The model under review builds one solid part; all positions refer to its coordinate system, in mm. Face numbers are marked on the shaded views. Give positions to 0.01 mm unless a question says otherwise; leave off trailing zeros. Loops run counter-clockwise (first coordinate to the right, second up) from the corner with the lowest first, then second, coordinate; pieces in that order, holes last. Notation, with made-up numbers: (43.5, -3.75) - (70.5, -3.75) arc R23 ccw to (70.5, 14.25) - close; hole circle Ø6 at (39, 7.25). An arc over 180 degrees is marked (long way). Return JSON: item names as keys, results as strings. Group by question number.
from build123d import *

# Parameters (mm, degrees)
BOSS_EXTRUDE2_DEPTH                        = 12.7
F_13_32_0_40625_DIAMETER_HOLE3_D           = 10.31875
F_13_32_0_40625_DIAMETER_HOLE3_CSINK_D     = 11.58875
F_13_32_0_40625_DIAMETER_HOLE3_CSINK_ANGLE = 90
F_13_32_0_40625_DIAMETER_HOLE2_D           = 10.31875
F_13_32_0_40625_DIAMETER_HOLE2_CSINK_D     = 11.58875
F_13_32_0_40625_DIAMETER_HOLE2_CSINK_ANGLE = 90


with BuildPart() as part:
    # Sketch1 → Boss-Extrude2 (new body)
    with BuildSketch(Plane(origin=(0, 0, 0), x_dir=(1, 0, 0), z_dir=(0, 1, 0))):
        with BuildLine():
            Line((0, 0), (101.6, 0))
            ThreePointArc((101.6, 0), (126.917817898, 23.358408246), (105.669972302, 50.471803395))
            Line((105.669972302, 50.471803395), (25.413803556, 63.5))
            Line((25.413803556, 63.5), (25.413803556, 76.2))
            Line((25.413803556, 76.2), (-25.386196444, 76.2))
            Line((-25.386196444, 76.2), (-25.386196444, 25.395653824))
            ThreePointArc((-25.386196444, 25.395653824), (-17.954095654, 7.438788683), (0, 0))
        make_face()
    extrude(amount=BOSS_EXTRUDE2_DEPTH)

    # 13/32 (0.40625) Diameter Hole3 (through all)
    with Locations(Plane(origin=(0, 12.7, 0), x_dir=(1, 0, 0), z_dir=(0, 1, 0))):
        with Locations((101.6, 25.4)):
            CounterSinkHole(F_13_32_0_40625_DIAMETER_HOLE3_D / 2, F_13_32_0_40625_DIAMETER_HOLE3_CSINK_D / 2, counter_sink_angle=F_13_32_0_40625_DIAMETER_HOLE3_CSINK_ANGLE)

    # 13/32 (0.40625) Diameter Hole2 (through all)
    with Locations(Plane(origin=(0, 12.7, 0), x_dir=(1, 0, 0), z_dir=(0, 1, 0))):
        with Locations((0, 25.386198205)):
            CounterSinkHole(F_13_32_0_40625_DIAMETER_HOLE2_D / 2, F_13_32_0_40625_DIAMETER_HOLE2_CSINK_D / 2, counter_sink_angle=F_13_32_0_40625_DIAMETER_HOLE2_CSINK_ANGLE)


solid = part.part
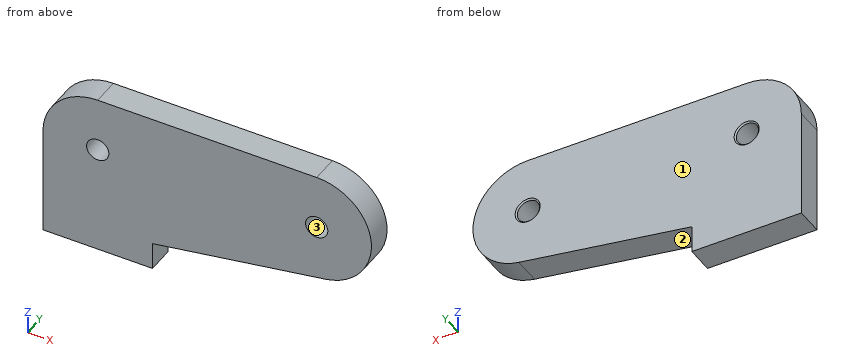
Item 1: For P1, Ø1.5, axis at x = 74.5, y = 6, coming from the -Z side; P2, Ø6, axis at x = 0, z = -25.39, coming from the -Y side; P3, Ø1, axis at y = 7, z = -14.5, coming from the -X side; P4, Ø1, axis at y = 3.5, z = -37, coming from the +X side, all flat-tipped, find the tip position at first contact; note any pin that passes through.
Item 2: Take a section at B-B (z = -58). State the section outline as (x, y) points.
Item 3: Take a section at A-A (y = 5.75). State the section outline as (x, z) points, then the cut area to 3 significant figures.
Item 4: Mouldability with a two-part tool opening along X and no side actions: class the marked faces 1, 2 and 3 as +X half, -X half, draft (parallel to the pull), parting line (faces both ways), or undercut.
Item 5: For L1, parallel to X at y = 4.75, z = -25.4; L2, parallel to X at y = 11.75, z = -22; L3, parallel to Z at x = 101.6, y = 4.5, list the stretches that pass through material, from the lowest coordinate up. Write a range as from..to.
Item 6: Take a section at C-C (x = 80). State the section outline as (y, z) points, then the cut area to 3 significant figures.
Check sheet entries:
{
 "1": {"P1": "stops at z = -55.65", "P2": "passes through", "P3": "stops at x = -23.16", "P4": "stops at x = 124.45"},
 "2": {"outline": "(-25.39, 0) - (59.29, 0) - (59.29, 12.7) - (-25.39, 12.7) - close"},
 "3": {"outline": "(-25.39, -76.2) - (25.41, -76.2) - (25.41, -63.5) - (105.67, -50.47) arc R25.4 ccw to (101.6, 0) - (0, 0) arc R25.39 ccw to (-25.39, -25.4) - close; hole circle Ø10.32 at (0, -25.39); hole circle Ø10.32 at (101.6, -25.4)", "area": "8,950 mm^2"},
 "4": {"face 1": "draft", "face 2": "+X half", "face 3": "undercut"},
 "5": {"L1": "x = -25.39..-5.16, 5.16..96.44, 106.76..127", "L2": "x = -25.16..-3.89, 3.89..97.72, 105.48..126.77", "L3": "z = -51.13..-30.56, -20.24..0"},
 "6": {"outline": "(0, -54.64) - (12.7, -54.64) - (12.7, 0) - (0, 0) - close", "area": "694 mm^2"}
}
